```python
from build123d import *
from build123d.topology import SkipClean

# Parameters (mm, degrees)
SKETCH_1_R          = 2
EXTRUDE_1_DEPTH     = 8
CUT_EXTRUDE_1_DEPTH = 2
EXTRUDE_START       = 4
SKETCH_4_3_R        = 2
EXTRUDE_2_DEPTH     = 4
FILLET_1_R          = 1.5


with BuildPart() as part:
    # Sketch 1 → Extrude 1 (new body)
    with BuildSketch(Plane.XY):
        with BuildLine():
            Line((-19.946933303, -8.027214437), (-17.618068878, -8.027214437))
            ThreePointArc((-17.618068878, -8.027214437), (-16.616104954, -8.139678872), (-15.664006617, -8.471475061))
            Line((-15.664006617, -8.471475061), (-10.511224254, -10.942177653))
            Line((-10.511224254, -10.942177653), (4, -10.942177653))
            ThreePointArc((4, -10.942177653), (5.414213562, -10.356391215), (6, -8.942177653))
            Line((6, -8.942177653), (6, 0))
            Line((6, 0), (6, 2.471508524))
            ThreePointArc((6, 2.471508524), (6.165879851, 3.269006662), (6.63600328, 3.934215927))
            Line((6.63600328, 3.934215927), (10.465403959, 7.505189831))
            ThreePointArc((10.465403959, 7.505189831), (10.846309641, 7.990494755), (11.061183494, 8.568801969))
            Line((11.061183494, 8.568801969), (13.877860093, 22.400226184))
            ThreePointArc((13.877860093, 22.400226184), (13.775141356, 22.81631716), (13.387916029, 23))
            Line((13.387916029, 23), (3.002563604, 23))
            ThreePointArc((3.002563604, 23), (2.686246444, 22.887225327), (2.51261954, 22.599773816))
            Line((2.51261954, 22.599773816), (0, 10.261436228))
            ThreePointArc((0, 10.261436228), (-1.001221601, 8.128058241), (-2.868431988, 6.690257248))
            Line((-2.868431988, 6.690257248), (-2.909187531, 6.672140294))
            ThreePointArc((-2.909187531, 6.672140294), (-4.995156756, 4.940562252), (-5.870795397, 2.374848493))
            Line((-5.870795397, 2.374848493), (-6, 0))
            Line((-6, 0), (-6, -4.601356756))
            Line((-6, -4.601356756), (-11, -4.329329712))
            Line((-11, -4.329329712), (-11, -2.078450028))
            Line((-11, -2.078450028), (-20.472837466, -1.563076433))
            ThreePointArc((-20.472837466, -1.563076433), (-20.84381589, -1.699308287), (-21, -2.062338084))
            Line((-21, -2.062338084), (-21, -5.795614421))
            Line((-21, -5.795614421), (-19.946933303, -8.027214437))
        make_face()
        Circle(SKETCH_1_R, mode=Mode.SUBTRACT)
    extrude(amount=EXTRUDE_1_DEPTH)

    # Sketch 4 → Cut-Extrude 1 (cut)
    with BuildSketch(Plane(origin=(0, 23, 0), x_dir=(1, 0, 0), z_dir=(0, 1, 0))):
        with BuildLine():
            ThreePointArc((11.195239817, -4), (9.16222587, -1.160116556), (5.818614501, -2.169248212))
            Line((5.818614501, -2.169248212), (6.61082294, -2.779498808))
            ThreePointArc((6.61082294, -2.779498808), (8.839897185, -2.106744371), (10.195239817, -4))
            ThreePointArc((10.195239817, -4), (10.088495446, -4.644657369), (9.779656693, -5.220501192))
            Line((9.779656693, -5.220501192), (10.571865132, -5.830751788))
            ThreePointArc((10.571865132, -5.830751788), (11.03512326, -4.966986053), (11.195239817, -4))
        make_face()
        with BuildLine():
            Line((6.61082294, -2.779498808), (5.818614501, -2.169248212))
            ThreePointArc((5.818614501, -2.169248212), (6.364488028, -6.376625315), (10.571865132, -5.830751788))
            Line((10.571865132, -5.830751788), (9.779656693, -5.220501192))
            ThreePointArc((9.779656693, -5.220501192), (6.974738624, -5.584416877), (6.61082294, -2.779498808))
        make_face()
    extrude(amount=-CUT_EXTRUDE_1_DEPTH, mode=Mode.SUBTRACT)

    # Sketch 4_3 → Extrude 2 (add)
    with SkipClean():  # the faces are left unmerged after this step: merging them gives an invalid solid
        with BuildSketch(Plane(origin=(0, 23, 0), x_dir=(1, 0, 0), z_dir=(0, 1, 0)).offset(EXTRUDE_START)):
            with Locations(Location((8.195239817, -4, 0), (0, 0, 270))):
                Circle(SKETCH_4_3_R)
        extrude(amount=-EXTRUDE_2_DEPTH)

    # Fillet 1
    fillet_1_edges = [part.edges().sort_by_distance(p)[0] for p in [
        (8.195239817, 27, 2),
    ]]
    fillet(fillet_1_edges, radius=FILLET_1_R)


solid = part.part
```
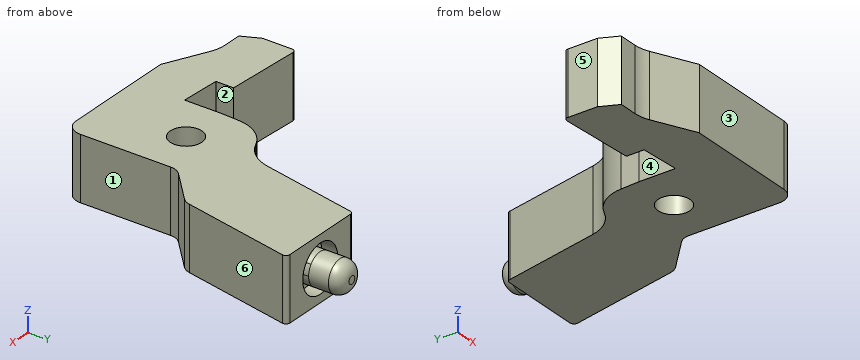
Input: part model. Units: mm. Frame: model coordinates. Face numbers are marked on the shaded views. A direction names the side the tool comes from. Give positions to 0.01 mm unless a question says otherwise; leave off trailing zeros. Loops run counter-clockwise (first coordinate to the right, second up) from the corner with the lowest first, then second, coordinate; pieces in that order, holes last. Notation, with made-up numbers: (89, 85) -> (135, 85) arc R23 ccw to (135, 109) -> close; hole circle Ø10 at (70, 66). An arc over 180 degrees is marked (long way). Use a Markdown table: item, result.
Q1. Access query for the marked faces 1, 2 and 3. Directions: +Z, -Z, +X, -X, +Y, -Y. A direction counts if a zero-diameter tool reaches every point of the face in a straight line with its end or side. Return the directions, or none.
Entries:
| item | result |
|---|---|
| face 1 | +Z, -Z, +X, -Y |
| face 2 | +Z, -Z, +Y |
| face 3 | +Z, -Z, +X, -X, -Y |
Q2. Pull-direction query (X, two-part tool) for the marked faces 4, 5 and 6; classes: pulls with the +X half, pulls with the -X half, needs draft (parallel to the pull), parting line crosses it, or undercut.
Entries:
| item | result |
|---|---|
| face 4 | undercut |
| face 5 | pulls with the -X half |
| face 6 | pulls with the +X half |
Q3. Section query A-A, the plane y = -2.5. Return the cut outline in (x, z).
Entries:
| item | result |
|---|---|
| outline | (-21, 0) -> (-11, 0) -> (-11, 8) -> (-21, 8) -> close; (-6, 0) -> (6, 0) -> (6, 8) -> (-6, 8) -> close |
Q4. Ray query, probe 1 along X at (y, z) = (-3, 1); probe 2 along X at (y, z) = (22, 6.75); probe 3 along Y at (x, z) = (-4.5, 5). Return the intervals inside material, ascending. Write a range as from..to.
Entries:
| item | result |
|---|---|
| probe 1 | x = -21..-11, -6..6 |
| probe 2 | x = 2.39..7, 9.39..13.8 |
| probe 3 | y = -10.94..5.55 |
Q5. Section query B-B, the plane x = -7. Return the cut outline in (y, z), plus the area to 3 significant figures.
Entries:
| item | result |
|---|---|
| outline | (-10.94, 0) -> (-4.55, 0) -> (-4.55, 8) -> (-10.94, 8) -> close |
| area | 51.2 mm² |
Q6. Section query C-C, the plane y = 18. Return the cut outline in (x, z).
Entries:
| item | result |
|---|---|
| outline | (1.58, 0) -> (12.98, 0) -> (12.98, 8) -> (1.58, 8) -> close |
Q7. First-contact query: P1, Ø5, axis at x = 0, y = 0, coming from the -Z side; P2, Ø1.2, axis at x = -18.5, z = 5, coming from the -Y side; P3, Ø1.5, axis at y = -5.5, z = 3, coming from the +X side; P4, Ø3, axis at x = -2, y = 11.5, coming from the +Z side. Flat tips, straight axial feed; report the tip coordinate or a pass-through.
Entries:
| item | result |
|---|---|
| P1 | stops at z = 0 |
| P2 | stops at y = -8.03 |
| P3 | stops at x = 6 |
| P4 | passes through |
